from build123d import *

# Parameters (mm, degrees)
F1_DEPTH = 12.7
F2_SIZE  = 15.24
F3_R     = 11.530279
F4_DEPTH = 12.7
F6_DEPTH = 63.5


with BuildPart() as f1:
    # F0 (on Top) → F1 (new body)
    with BuildSketch(Plane.XY):
        Polygon((28.575, 28.575), (0, 28.575), (-28.575, 28.575), (-28.575, 0), (-28.575, -28.575), (0, -28.575), (28.575, -28.575), (28.575, 0), align=None)
    extrude(amount=F1_DEPTH)

    # F2
    f2_edges = [f1.edges().sort_by_distance(p)[0] for p in [
        (28.575, -28.575, 6.35),
        (-28.575, -28.575, 6.35),
    ]]
    chamfer(f2_edges, length=F2_SIZE)

    # F3 (on face) → F4 (cut)
    with BuildSketch(Plane.XY.offset(12.7)):
        with Locations((0, -13.289176)):
            Circle(F3_R)
    extrude(amount=-F4_DEPTH, mode=Mode.SUBTRACT)

    # F5 (on face) → F6 (cut)
    with BuildSketch(Plane.YZ.offset(28.575)):
        with BuildLine():
            Line((23.010647, 12.7), (1.922707, 12.7))
            ThreePointArc((1.922707, 12.7), (12.466677, 2.15603), (23.010647, 12.7))
        make_face()
    extrude(amount=-F6_DEPTH, mode=Mode.SUBTRACT)


solid = f1.part
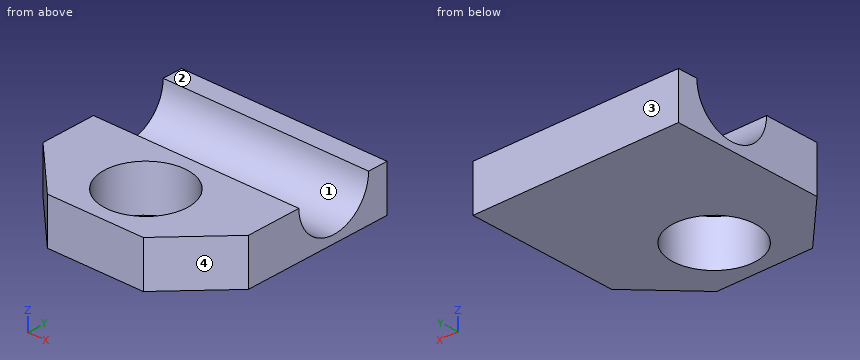
The listing builds one solid part. Answer for the finished solid, in the listing's coordinates (mm). Face numbers are marked on the shaded views. Coordinates: 2 decimals unless noted, no trailing zeros. Loops run counter-clockwise (first coordinate to the right, second up) from the corner with the lowest first, then second, coordinate; pieces in that order, holes last. Notation, with made-up numbers: (0, 65) -> (49, 65) arc R4 ccw to (49, 71) -> close; hole circle Ø4 at (26, -4). An arc over 180 degrees is marked (long way). Answer in a Markdown table with one row per item. Add a question column.
1. A flat-ended cylindrical pin translates along its axis: P1, Ø1.5, axis at y = 21, z = 9.5, coming from the -X side. Find the tip coordinate at first contact, or state that the pin passes through.
2. The part is cut by section B-B, the plane z = 5. Write down the section's boundary in (x, y) (3 decimals).
3. Determine the mould class of the marked faces 1, 2, 3 and 4 for opening direction Y: +Y half, -Y half, draft (parallel to the pull), parting line (faces both ways), or undercut.
4. The part is cut by section D-D, the plane x = 16. Write down the section's boundary in (y, z) (3 decimals).
5. Consider line 1 (Y direction, x = -9.5, z = 7.25) (1 decimal); line 2 (Y direction, x = -3.5, z = 5.75) (3 decimals); line 3 (X direction, y = -4, z = 0.5) (3 decimals). Determine where each line is inside the solid, lowest interval first. Write a range as [from, to].
6. The part is cut by section A-A, the plane x = 0. Write down the section's boundary in (y, z) (3 decimals).
7. The part is cut by section C-C, the plane y = -9.5. Write down the section's boundary in (x, z) (3 decimals), then the cut area to 3 significant figures.
Answer below:
| question | item | result |
|---|---|---|
| 1 | P1 | through |
| 2 | outline | (-28.575, -13.335) -> (-13.335, -28.575) -> (13.335, -28.575) -> (28.575, -13.335) -> (28.575, 5.264) -> (-28.575, 5.264) -> close; (-28.575, 19.67) -> (28.575, 19.67) -> (28.575, 28.575) -> (-28.575, 28.575) -> close; hole circle Ø23.061 at (0, -13.289) |
| 3 | face 1 | undercut |
| 3 | face 2 | draft |
| 3 | face 3 | +Y half |
| 3 | face 4 | -Y half |
| 4 | outline | (-25.91, 0) -> (28.575, 0) -> (28.575, 12.7) -> (23.011, 12.7) arc R10.544 cw to (1.923, 12.7) -> (-25.91, 12.7) -> close |
| 5 | line 1 | [-28.6, -19.8], [-6.8, 3.4], [21.5, 28.6] |
| 5 | line 2 | [-28.575, -24.275], [-2.303, 4.537], [20.396, 28.575] |
| 5 | line 3 | [-28.575, -6.831], [6.831, 28.575] |
| 6 | outline | (-28.575, 0) -> (-24.819, 0) -> (-24.819, 12.7) -> (-28.575, 12.7) -> close; (-1.759, 0) -> (28.575, 0) -> (28.575, 12.7) -> (23.011, 12.7) arc R10.544 cw to (1.923, 12.7) -> (-1.759, 12.7) -> close |
| 7 | outline | (-28.575, 0) -> (-10.89, 0) -> (-10.89, 12.7) -> (-28.575, 12.7) -> close; (10.89, 0) -> (28.575, 0) -> (28.575, 12.7) -> (10.89, 12.7) -> close |
| 7 | area | 449 mm2 |
